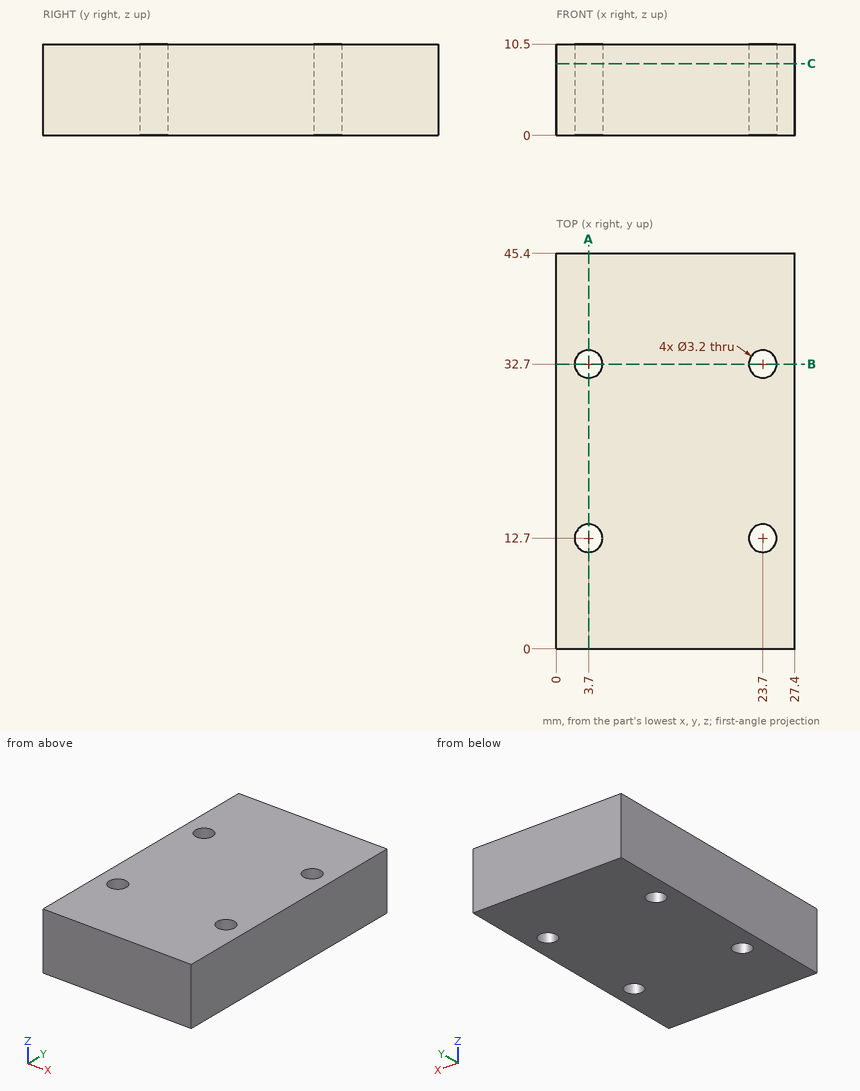
Study the drawing (mm; zero at the part's minimum x, y, z) and answer. Give positions to 0.01 mm unless a question says otherwise; leave off trailing zeros. Loops run counter-clockwise (first coordinate to the right, second up) from the corner with the lowest first, then second, coordinate; pieces in that order, holes last. Notation, with made-up numbers: (26.25, 88.5) -> (53.25, 88.5) arc R18 ccw to (53.25, 99.5) -> close; hole circle Ø2 at (8.5, 49.5). An arc over 180 degrees is marked (long way). Write item = value, one per line. Start each with the question number.
(1) Find the intervals of material crossed by probe 1 along X at (y, z) = (32.7, 8.5); probe 2 along Y at (x, z) = (23.7, 4); probe 3 along Y at (x, z) = (4.25, 2), in increasing order. Write a range as from..to.
(2) Find section A-A on x = 3.7. Give the vertices of the cut face in (y, z).
(3) Given pin 1 Ø3 at (x, y) = (3.7, 32.7) entering from +Z (3 decimals), flat-ended and moving along its own axis, determine where the tip first touches the part or whether it passes through.
(4) Find section C-C on z = 8.25. Give the vertices of the cut face in (x, y).
(5) Find section B-B on y = 32.7. Give the vertices of the cut face in (x, z), and give its area (4 significant figures).
From the geometry:
q1.probe_1 = 0..2.1, 5.3..22.1, 25.3..27.4
q1.probe_2 = 0..11.1, 14.3..31.1, 34.3..45.4
q1.probe_3 = 0..11.2, 14.2..31.2, 34.2..45.4
q2.outline = (0, 0) -> (11.1, 0) -> (11.1, 10.5) -> (0, 10.5) -> close; (14.3, 0) -> (31.1, 0) -> (31.1, 10.5) -> (14.3, 10.5) -> close; (34.3, 0) -> (45.4, 0) -> (45.4, 10.5) -> (34.3, 10.5) -> close
q3.pin_1 = through
q4.outline = (0, 0) -> (27.4, 0) -> (27.4, 45.4) -> (0, 45.4) -> close; hole circle Ø3.2 at (3.7, 12.7); hole circle Ø3.2 at (3.7, 32.7); hole circle Ø3.2 at (23.7, 12.7); hole circle Ø3.2 at (23.7, 32.7)
q5.outline = (0, 0) -> (2.1, 0) -> (2.1, 10.5) -> (0, 10.5) -> close; (5.3, 0) -> (22.1, 0) -> (22.1, 10.5) -> (5.3, 10.5) -> close; (25.3, 0) -> (27.4, 0) -> (27.4, 10.5) -> (25.3, 10.5) -> close
q5.area = 220.5 mm^2
